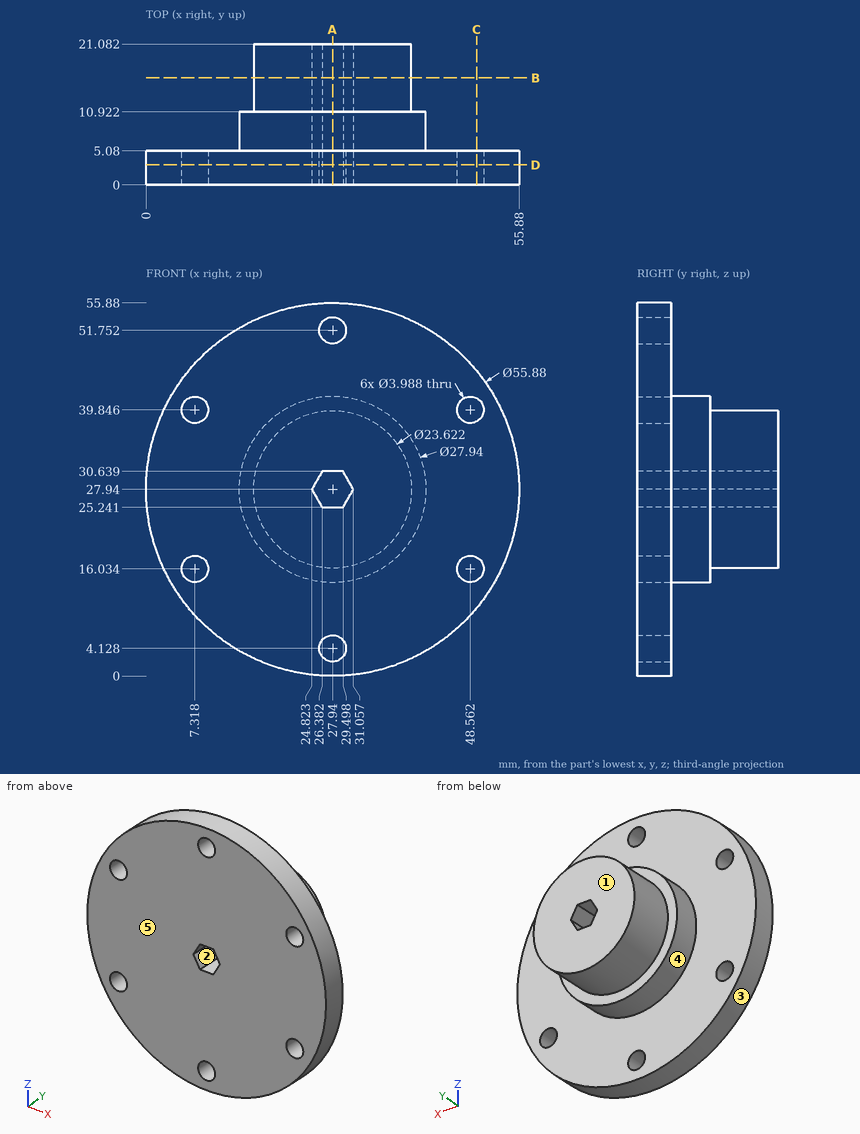
Source: three-view drawing plus pictorial views. Frame: mm from the lowest corner of the part. A direction names the side the tool comes from. Give positions to 0.01 mm unless a question says otherwise; leave off trailing zeros. Write each loop counter-clockwise with the first axis right and the second up, starting at its lowest first coordinate (ties: lowest second). Pieces come first, ordered by that corner, then holes.
(1) Ray query, line 1 (Z direction, x = 27.94, y = 3.3); line 2 (Y direction, x = 5, z = 18.5); line 3 (Z direction, x = 8, y = 5) (1 decimal). Return the intervals inside material, ascending.
(2) Cut plane D-D, the plane y = 3. Return loops of the section in (x, z), then the cut area to 3 significant figures.
(3) Cut plane C-C, the plane x = 49.5. Return loops of the section in (y, z) (1 decimal), then the cut area to 3 significant figures.
(4) First-contact query: P1, Ø3, axis at x = 18, y = 8.5, coming from the +Z side; P2, Ø2, axis at x = 18.5, y = 5.5, coming from the -Z side (1 decimal); P3, Ø5, axis at x = 7.32, z = 16.03, coming from the +Y side. Flat tips, straight axial feed; report the tip coordinate or a pass-through.
(5) Access query for the marked faces 4 and 5. Directions: +Z, -Z, +X, -X, +Y, -Y. A direction counts if a zero-diameter tool reaches every point of the face in a straight line with its end or side. Return the directions, or none.
(6) Cut plane A-A, the plane x = 27.94. Return loops of the section in (y, z).
(7) Mould query, pull axis Z, two halves, no side actions, for the marked faces 1, 2 and 3. Classes: released by +Z, released by -Z, zero draft, split by the parting line, or undercut.
(8) Cut plane B-B, the plane y = 16. Return loops of the section in (x, z).
Values follow:
1. line 1: z = 0 to 2.13, 6.12 to 25.24, 30.64 to 49.76, 53.75 to 55.88
1. line 2: y = 0 to 5.08
1. line 3: z = 8.4 to 14.2, 17.9 to 38, 41.7 to 47.5
2. outline: circle Ø55.88 at (27.94, 27.94); hole circle Ø3.99 at (7.32, 16.03); hole circle Ø3.99 at (7.32, 39.85); hole (24.82, 27.94) - (26.38, 25.24) - (29.5, 25.24) - (31.06, 27.94) - (29.5, 30.64) - (26.38, 30.64) - close; hole circle Ø3.99 at (27.94, 4.13); hole circle Ø3.99 at (27.94, 51.75); hole circle Ø3.99 at (48.56, 16.03); hole circle Ø3.99 at (48.56, 39.85)
2. area: 2,350 mm2
3. outline: (0, 10.2) - (5.1, 10.2) - (5.1, 14.3) - (0, 14.3) - close; (0, 17.8) - (5.1, 17.8) - (5.1, 38.1) - (0, 38.1) - close; (0, 41.6) - (5.1, 41.6) - (5.1, 45.7) - (0, 45.7) - close
3. area: 145 mm2
4. P1: stops at z = 39.07
4. P2: stops at z = 1.3
4. P3: stops at y = 5.08
5. face 4: +Y
5. face 5: +Z, -Z, +X, -X, -Y
6. outline: (0, 0) - (5.08, 0) - (5.08, 2.13) - (0, 2.13) - close; (0, 6.12) - (5.08, 6.12) - (5.08, 13.97) - (10.92, 13.97) - (10.92, 16.13) - (21.08, 16.13) - (21.08, 25.24) - (0, 25.24) - close; (0, 30.64) - (21.08, 30.64) - (21.08, 39.75) - (10.92, 39.75) - (10.92, 41.91) - (5.08, 41.91) - (5.08, 49.76) - (0, 49.76) - close; (0, 53.75) - (5.08, 53.75) - (5.08, 55.88) - (0, 55.88) - close
7. face 1: zero draft
7. face 2: undercut
7. face 3: split by the parting line
8. outline: circle Ø23.62 at (27.94, 27.94); hole (24.82, 27.94) - (26.38, 25.24) - (29.5, 25.24) - (31.06, 27.94) - (29.5, 30.64) - (26.38, 30.64) - close
